from build123d import *

# Parameters (mm, degrees)
SKETCH_1_W      = 5
SKETCH_1_H      = 5
EXTRUDE_1_DEPTH = 24
CHAMFER_1_SIZE  = 5


with BuildPart() as part:
    # ｽｹｯﾁ1 → ﾎﾞｽ - 押し出し1 (new body)
    with BuildSketch(Plane.XY):
        with Locations((2.5, 2.5)):
            Rectangle(SKETCH_1_W, SKETCH_1_H)
    extrude(amount=EXTRUDE_1_DEPTH)

    # 面取り1
    chamfer_1_edges = [part.edges().sort_by_distance(p)[0] for p in [
        (5, 5, 12),
    ]]
    chamfer(chamfer_1_edges, length=CHAMFER_1_SIZE - 0.0001)  # a hair under: the kernel refuses the full size


solid = part.part
Read the model definition and answer for the solid it produces. Units are mm, in the model's axes. Coordinates: 2 decimals unless noted, no trailing zeros. Order: outer loops, then holes, each group sorted by start corner. A loop starts at its lowest first (then second) coordinate and runs counter-clockwise, first axis right, second up. Notation, with made-up numbers: M -5,5.25 L 16,5.25 A11 cw 16,12.25 Z; hole C 8,18 d7. An arc over 180 degrees is marked long. Put each result on its own line as item: value. Start each with the question number.
Item 1: Given pin 1 Ø2 at (y, z) = (2.5, 13) entering from +X, flat-ended and moving along its own axis, determine where the tip first touches the part or whether it passes through.
Item 2: Consider probe 1 along X at (y, z) = (0.4, 8.75); probe 2 along Y at (x, z) = (2, 16); probe 3 along Y at (x, z) = (1.25, 11.25). Determine where each line is inside the solid, lowest interval first. Write a range as [from, to].
Item 3: Section B-B, the plane y = 3.8 is taken. Determine the outline of the cut face in (x, z).
Item 4: The mould has two halves that part along Y. Classify faces 1 (the face through (2, 0, 12)), 2 (the face through (2, 2, 24)), 3 (the face through (2, 3, 12)): +Y half, -Y half, draft (parallel to the pull), parting line (faces both ways), or undercut.
Item 5: Section C-C, the plane x = 4.4 is taken. Determine the outline of the cut face in (y, z).
Computed:
1. pin 1: stops at x = 3.5
2. probe 1: x = [0, 4.6]
2. probe 2: y = [0, 3]
2. probe 3: y = [0, 3.75]
3. outline: M 0,0 L 1.2,0 L 1.2,24 L 0,24 Z
4. face 1: -Y half
4. face 2: draft
4. face 3: +Y half
5. outline: M 0,0 L 0.6,0 L 0.6,24 L 0,24 Z
